Could you check a few things on this model? Use its own coordinates, in mm. A direction names the side the tool comes from. Coordinates: 2 decimals unless noted, no trailing zeros. Loops run counter-clockwise (first coordinate to the right, second up) from the corner with the lowest first, then second, coordinate; pieces in that order, holes last.
from build123d import *

# Parameters (mm, degrees)
F1_DEPTH = 76.2
F3_DEPTH = 38.1


with BuildPart() as f1:
    # F0 (on Top) → F1 (new body)
    with BuildSketch(Plane.XY):
        Polygon((-19.342009, 43.308758), (-57.442009, 43.308758), (-57.442009, -32.891242), (56.857991, -32.891242), (56.857991, 43.308758), (18.757991, 43.308758), (18.757991, 5.208758), (-19.342009, 5.208758), align=None)
    extrude(amount=-F1_DEPTH)

    # F2 (on face) → F3 (cut)
    with BuildSketch(Plane(origin=(0, 43.308758, 0), x_dir=(-1, 0, 0), z_dir=(0, 1, 0))):
        Polygon((-18.757991, -50.457798), (-18.757991, -33.375844), (-56.857991, -33.375844), (-56.857991, -34.49871), (-56.857991, -50.457798), align=None)
    extrude(amount=-F3_DEPTH, mode=Mode.SUBTRACT)


solid = f1.part
(1) We'd pull the mould along X, two halves only. Please class faces 4 (the face through (38, 25, -50.458)), 5 (the face through (-19.342, 24, -38)), 6 (the face through (-57.442, 6, -38)), 7 (the face through (18.758, 25, -16)): +X half, -X half, draft (parallel to the pull), parting line (faces both ways), or undercut.
Answers:
face 4: draft
face 5: undercut
face 6: -X half
face 7: undercut
(2) For pin 1 (10 mm diameter, centred on x = -11.5, z = -42, fed in from +Y), with a flat end and sliding along its axis, tell me the tip position at first contact or that it passes through.
Answers:
pin 1: stops at y = 5.21
(3) Imagine slicing it at B-B, the plane x = 50.5. Write out the boundary of the cut face in (y, z).
Answers:
outline: (-32.89, -76.2) - (43.31, -76.2) - (43.31, -50.46) - (5.21, -50.46) - (5.21, -33.38) - (43.31, -33.38) - (43.31, 0) - (-32.89, 0) - close
(4) Imagine slicing it at C-C, the plane z = -43. Write out the boundary of the cut face in (x, y).
Answers:
outline: (-57.44, -32.89) - (56.86, -32.89) - (56.86, 5.21) - (-19.34, 5.21) - (-19.34, 43.31) - (-57.44, 43.31) - close
(5) Imagine slicing it at D-D, the plane z = -57. Write out the boundary of the cut face in (x, y), and give its area (3 significant figures).
Answers:
outline: (-57.44, -32.89) - (56.86, -32.89) - (56.86, 43.31) - (18.76, 43.31) - (18.76, 5.21) - (-19.34, 5.21) - (-19.34, 43.31) - (-57.44, 43.31) - close
area: 7,260 mm2
(6) Which directions (+Z, -Z, +X, -X, +Y, -Y) give clear straight access to the entire face, cutting with the end or side of a thin tool? Please do faces 1 (the face through (18.758, 25, -63)), 2 (the face through (38, 43.309, -16)), 3 (the face through (38, 25, -33.376)).
Answers:
face 1: +Z, -Z, +Y
face 2: +Z, -Z, +X, -X, +Y
face 3: +X, +Y
(7) I need wall thicknesses on probe 1 along X at (y, z) = (17.5, -60.5); probe 2 along Z at (x, y) = (35, 24); probe 3 along Y at (x, z) = (-18, -26). Which ranges of each line are inside material? Lowest first, please.
Answers:
probe 1: x = -57.44 to -19.34, 18.76 to 56.86
probe 2: z = -76.2 to -50.46, -33.38 to 0
probe 3: y = -32.89 to 5.21
(8) Imagine slicing it at A-A, the plane y = 14. Write out the boundary of the cut face in (x, z), and give its area (3 significant figures).
Answers:
outline: (-57.44, -76.2) - (-19.34, -76.2) - (-19.34, 0) - (-57.44, 0) - close; (18.76, -76.2) - (56.86, -76.2) - (56.86, -50.46) - (18.76, -50.46) - close; (18.76, -33.38) - (56.86, -33.38) - (56.86, 0) - (18.76, 0) - close
area: 5,160 mm2
